Here's the drawing with two shaded views (mm, measured from the low corner). I have some questions. A direction names the side the tool comes from. Coordinates: 2 decimals unless noted, no trailing zeros. Order: outer loops, then holes, each group sorted by start corner. A loop starts at its lowest first (then second) coordinate and runs counter-clockwise, first axis right, second up. Notation, with made-up numbers: (0.5, 82.5) - (40.5, 82.5) arc R12 ccw to (40.5, 96.5) - close; hole circle Ø5 at (-15, -18). An arc over 180 degrees is marked (long way). Answer as CSV lines item,"result". Start each with the question number.
1. I want a section at A-A, the plane z = 15.24. List the corners of the cut face in (x, y) for me.
2. For pin 1 (0.8 mm diameter, centred on x = 15, y = 1.5, fed in from -Z); pin 2 (4.5 mm diameter, centred on x = 21.209, y = 9.779, fed in from -Z); pin 3 (5 mm diameter, centred on x = 12, y = 19.5, fed in from +Z); pin 4 (4 mm diameter, centred on x = 11.5, z = 11.5, fed in from +Y), each with a flat end and sliding along its axis, tell me the tip position at first contact or that it passes through.
3. I want a section at B-B, the plane x = 17. List the corners of the cut face in (y, z) for me (3 decimals).
4. I need wall thicknesses on probe 1 along Z at (x, y) = (3.75, 2); probe 2 along X at (y, z) = (1.05, 15.24); probe 3 along Y at (x, z) = (20.75, 7.25). Which ranges of each line are inside material? Lowest first, please.
5. For the marked faces 1 and 2, which set-ups out of +Z, -Z, +X, -X, +Y, -Y let a thin tool reach every point of the face, with its end or its side?
6. I want a section at C-C, the plane y = 4. List the corners of the cut face in (x, z) for me.
7. I want a section at D-D, the plane x = 21.59. List the corners of the cut face in (y, z) for me, and give its area (3 significant figures).
8. Thinking about a two-plate mould opening in Z: for the marked faces 3, 4 and 5, which applies, released by +Z, released by -Z, zero draft, split by the parting line, or undercut?
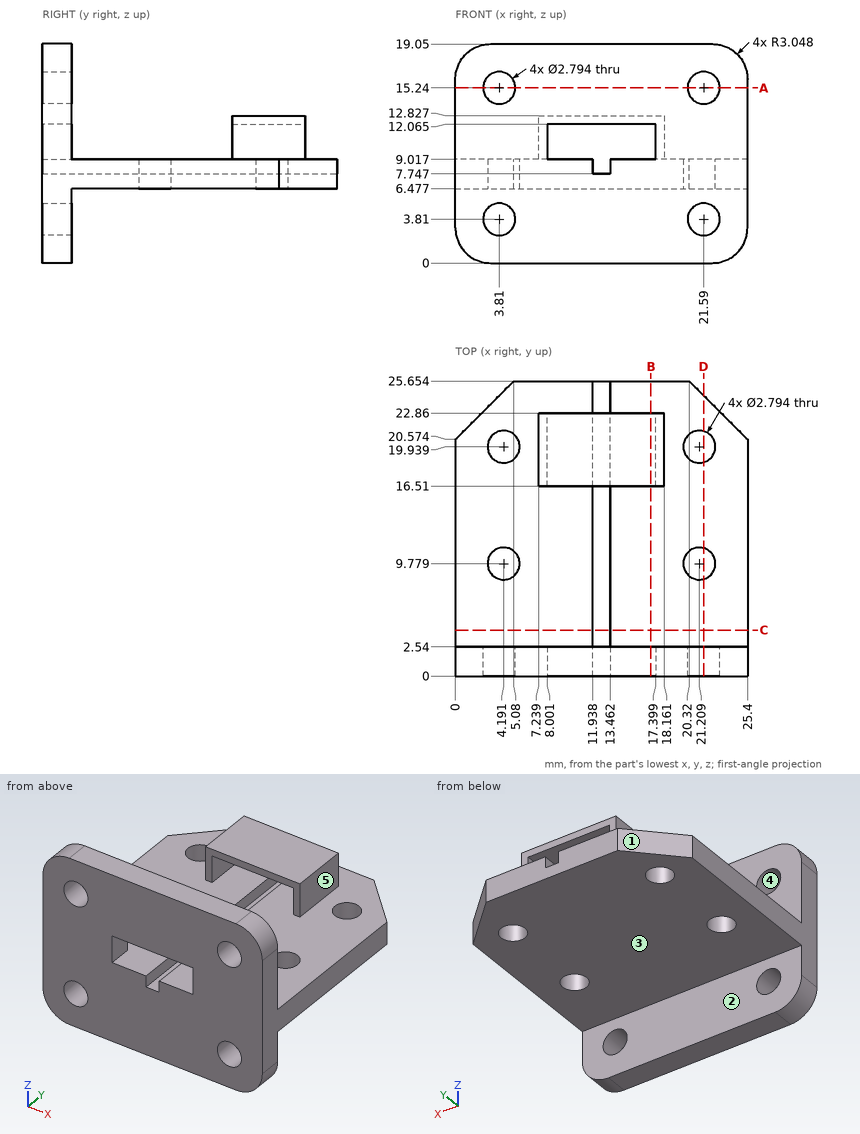
Solved:
1,outline,"(0, 0) - (2.41, 0) - (2.41, 2.54) - (0, 2.54) - close; (5.21, 0) - (20.19, 0) - (20.19, 2.54) - (5.21, 2.54) - close; (22.99, 0) - (25.4, 0) - (25.4, 2.54) - (22.99, 2.54) - close"
2,pin 1,"stops at z = 0"
2,pin 2,"stops at z = 6.48"
2,pin 3,"stops at z = 12.83"
2,pin 4,"stops at y = 22.86"
3,outline,"(0, 0) - (2.54, 0) - (2.54, 6.477) - (25.654, 6.477) - (25.654, 9.017) - (0, 9.017) - close; (0, 12.065) - (2.54, 12.065) - (2.54, 19.05) - (0, 19.05) - close; (16.51, 12.065) - (22.86, 12.065) - (22.86, 12.827) - (16.51, 12.827) - close"
4,probe 1,"z = 0 to 2.41, 5.21 to 13.84, 16.64 to 19.05"
4,probe 2,"x = 0 to 2.41, 5.21 to 20.19, 22.99 to 25.4"
4,probe 3,"y = 0 to 8.46, 11.1 to 18.62, 21.26 to 25.22"
5,face 1,"+Z, -Z, -X, +Y"
5,face 2,"-Z, +X, -X, +Y"
6,outline,"(0, 6.48) - (25.4, 6.48) - (25.4, 9.02) - (13.46, 9.02) - (13.46, 7.75) - (11.94, 7.75) - (11.94, 9.02) - (0, 9.02) - close"
7,outline,"(0, 0) - (2.54, 0) - (2.54, 2.41) - (0, 2.41) - close; (0, 5.21) - (2.54, 5.21) - (2.54, 6.48) - (8.43, 6.48) - (8.43, 9.02) - (2.54, 9.02) - (2.54, 13.84) - (0, 13.84) - close; (0, 16.64) - (2.54, 16.64) - (2.54, 19.05) - (0, 19.05) - close; (11.12, 6.48) - (18.59, 6.48) - (18.59, 9.02) - (11.12, 9.02) - close; (21.28, 6.48) - (24.38, 6.48) - (24.38, 9.02) - (21.28, 9.02) - close"
7,area,"76.0 mm2"
8,face 3,"released by -Z"
8,face 4,"undercut"
8,face 5,"zero draft"
